Here's how the part is built. I have some questions about the finished solid (model axes, mm). A direction names the side the tool comes from. Round coordinates to 2 decimals unless told otherwise and drop trailing zeros. Write each loop counter-clockwise with the first axis right and the second up, starting at its lowest first coordinate (ties: lowest second). Pieces come first, ordered by that corner, then holes. Notation, with made-up numbers: (89.25, 2) - (115.25, 2) arc R19 ccw to (115.25, 26) - close; hole circle Ø5 at (51, -12.75). An arc over 180 degrees is marked (long way). Use one line per item in the form item = value. Start each with the question number.
1. If I drill on line 1 along Z through (x, y) = (1.75, 3.5); line 2 along Z through (x, y) = (-1, 2.75); line 3 along Z through (x, y) = (3, 6.25), over which ranges is the centre line in solid material (lowest first)?
2. I want a section at B-B, the plane z = -37. List the corners of the cut face in (x, y) for me, plus the area to 3 significant figures.
3. Which directions (+Z, -Z, +X, -X, +Y, -Y) give clear straight access to the entire face, cutting with the end or side of a thin tool? Please do faces 4 (the cylindrical face through (-0.046, -9.525, -11.823)), 5 (the cylindrical face through (-2.33, -0.31, -6.29)), 6 (the cylindrical face through (1.26, 3.05, -55.58)).
4. Will these pins go through, and if not, where does the flat tip stop? pin 1 (5 mm diameter, centred on y = -2.5, z = -39.5, fed in from +X); pin 2 (3 mm diameter, centred on y = 3.5, z = -50.5, fed in from -X).
5. We'd pull the mould along Z, two halves only. Please class faces 1 (the flat face through (-1.2, 2.2, -1.524)), 2 (the cylindrical face through (-5.037, -0.661, -0.773)), 3 (the flat face through (-4, 0, -12.7)): +Z half, -Z half, draft (parallel to the pull), parting line (faces both ways), or undercut.
6. I want a section at A-A, the plane x = 0. List the corners of the cut face in (y, z) for me (1 decimal).
```python
from build123d import *

# Parameters (mm, degrees)
CORTAR_EXTRUIR1_START = -1.778
CORTAR_EXTRUIR1_DEPTH = 1.778


# Read off the part's stored shape, not the designer's step: Cortar-Extruir1
with BuildPart() as part:
    # Croquis1 → Revolución1 (revolve)
    with BuildSketch(Plane(origin=(0, 0, 0), x_dir=(0, 0, -1), z_dir=(1, 0, 0))):
        Polygon((0, 0), (0, 5.08), (1.524, 5.08), (1.524, 2.3495), (10.922, 2.3495), (10.922, 9.525), (12.7, 9.525), (12.7, 3.302), (97.282, 3.302), (97.282, 0), align=None)
    revolve(axis=Axis((0, 0, -97.282), (0, 0, 1)))

    # Cortar-Extruir1 outline → Cortar-Extruir1 (cut)
    with BuildSketch(Plane.XY.offset(-10.922).offset(CORTAR_EXTRUIR1_START)):
        with BuildLine():
            Line((-3.25214663, -8.952606732), (-5.207, 0))
            Line((-5.207, 0), (-3.25214663, 8.952606732))
            ThreePointArc((-3.25214663, 8.952606732), (-9.525, 0), (-3.25214663, -8.952606732))
        make_face()
        with BuildLine():
            Line((5.207, 0), (3.25214663, -8.952606732))
            ThreePointArc((3.25214663, -8.952606732), (9.525, 0), (3.25214663, 8.952606732))
            Line((3.25214663, 8.952606732), (5.207, 0))
        make_face()
    extrude(amount=CORTAR_EXTRUIR1_DEPTH, mode=Mode.SUBTRACT)


solid = part.part
```
Model answer:
q1.line_1 = -12.7 to -10.92, -1.52 to 0
q1.line_2 = -97.28 to -10.92, -1.52 to 0
q1.line_3 = -12.7 to -10.92
q2.outline = circle Ø6.6 at (0, 0)
q2.area = 34.3 mm2
q3.face_4 = +Z, -Z, -Y
q3.face_5 = none
q3.face_6 = -Z
q4.pin_1 = 3.3
q4.pin_2 = -2.63
q5.face_1 = undercut
q5.face_2 = draft
q5.face_3 = -Z half
q6.outline = (-9.5, -12.7) - (-3.3, -12.7) - (-3.3, -97.3) - (3.3, -97.3) - (3.3, -12.7) - (9.5, -12.7) - (9.5, -10.9) - (2.3, -10.9) - (2.3, -1.5) - (5.1, -1.5) - (5.1, 0) - (-5.1, 0) - (-5.1, -1.5) - (-2.3, -1.5) - (-2.3, -10.9) - (-9.5, -10.9) - close
